Source: three-view drawing plus pictorial views. Frame: mm from the lowest corner of the part. A direction names the side the tool comes from. Round coordinates to 2 decimals unless told otherwise and drop trailing zeros. Loops run counter-clockwise (first coordinate to the right, second up) from the corner with the lowest first, then second, coordinate; pieces in that order, holes last. Notation, with made-up numbers: M 39,57 L 71,57 A13 ccw 71,82 Z; hole C 21.5,19.5 d6. An arc over 180 degrees is marked long. Return JSON: item names as keys, results as strings. Group by question number.
1) Material intervals for line 1 (X direction, y = 15.25, z = 11) (1 decimal); line 2 (Y direction, x = 28.5, z = 9.5); line 3 (Z direction, x = 14.5, y = 16.25), sorted ascending. Write a range as from..to.
2) Access query for the marked faces 4, 5, 6, 7 and 8. Directions: +Z, -Z, +X, -X, +Y, -Y. A direction counts if a zero-diameter tool reaches every point of the face in a straight line with its end or side. Return the directions, or none.
3) Section C-C (x = 7.5). Output: boundary loops of the cut face in (y, z).
4) Section A-A (z = 11). Output: boundary loops of the cut face in (x, y) (1 decimal), plus the area to 3 significant figures.
5) Section D-D (y = 8.75). Output: boundary loops of the cut face in (x, z) (1 decimal), plus the area to 3 significant figures.
6) Section B-B (z = 2.5). Output: boundary loops of the cut face in (x, y) (1 decimal), plus the area to 3 significant figures.
7) Contact query for flat-ended pins moving along their axis: P1, Ø9, axis at x = 24.74, z = 11, coming from the -Y side; P2, Ø5.5, axis at y = 17, z = 20, coming from the +X side; P3, Ø2, axis at y = 11.5, z = 20, coming from the -X side; P4, Ø1.5, axis at x = 43.5, z = 9, coming from the -Y side. Output: stop coordinate, or through.
8) Mould query, pull axis X, two halves, no side actions, for the marked faces 1, 2 and 3. Classes: +X half, -X half, draft (parallel to the pull), parting line (faces both ways), or undercut.
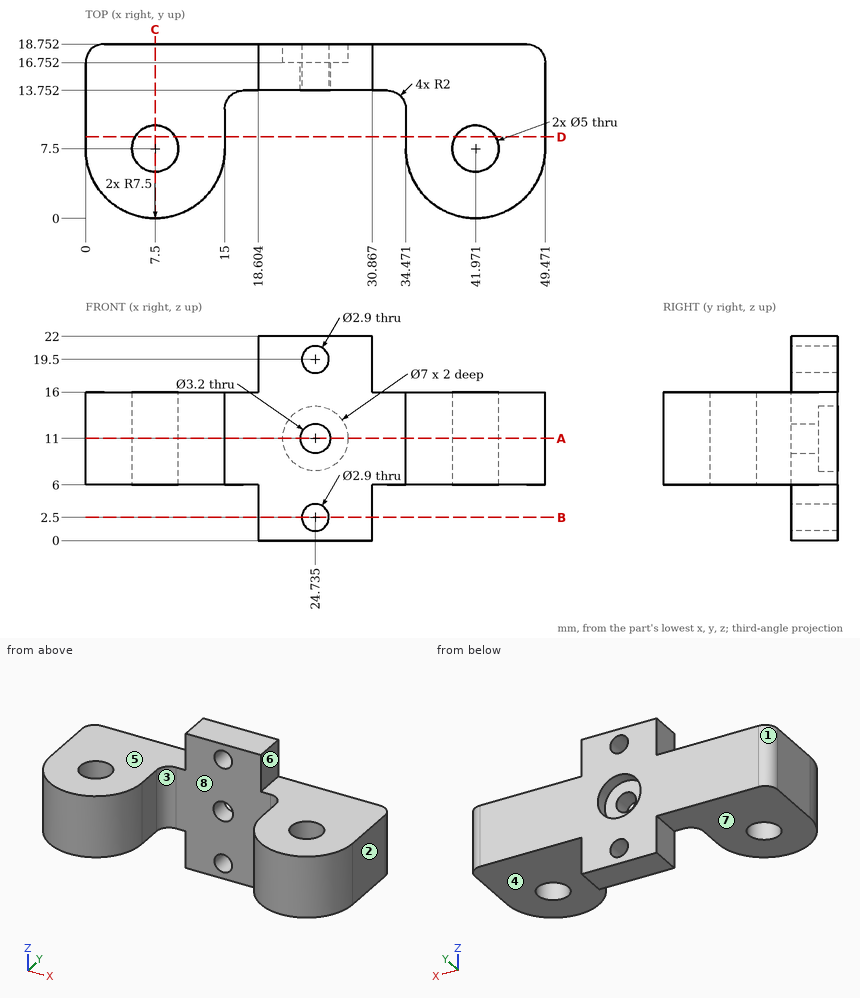
Returned:
{
 "1": {"line 1": "x = 0..23.1, 26.3..49.5", "line 2": "y = 13.75..18.75", "line 3": "z = 6..16"},
 "2": {"face 4": "-Z, +X, +Y, -Y", "face 5": "+Z, -X, +Y, -Y", "face 6": "+Z, +X, +Y, -Y", "face 7": "-Z, -X, +Y, -Y", "face 8": "+Z, -Z, -Y"},
 "3": {"outline": "M 0,6 L 5,6 L 5,16 L 0,16 Z; M 10,6 L 18.75,6 L 18.75,16 L 10,16 Z"},
 "4": {"outline": "M 0,7.5 A7.5 ccw 15,7.5 L 15,11.8 A2 cw 17,13.8 L 23.1,13.8 L 23.1,16.8 L 21.2,16.8 L 21.2,18.8 L 2,18.8 A2 ccw 0,16.8 Z; M 26.3,13.8 L 32.5,13.8 A2 cw 34.5,11.8 L 34.5,7.5 A7.5 ccw 49.5,7.5 L 49.5,16.8 A2 ccw 47.5,18.8 L 28.2,18.8 L 28.2,16.8 L 26.3,16.8 Z; hole C 7.5,7.5 d5; hole C 42,7.5 d5", "area": "549 mm^2"},
 "5": {"outline": "M 0,6 L 5.3,6 L 5.3,16 L 0,16 Z; M 9.7,6 L 15,6 L 15,16 L 9.7,16 Z; M 34.5,6 L 39.8,6 L 39.8,16 L 34.5,16 Z; M 44.1,6 L 49.5,6 L 49.5,16 L 44.1,16 Z", "area": "213 mm^2"},
 "6": {"outline": "M 18.6,13.8 L 23.3,13.8 L 23.3,18.8 L 18.6,18.8 Z; M 26.2,13.8 L 30.9,13.8 L 30.9,18.8 L 26.2,18.8 Z", "area": "46.8 mm^2"},
 "7": {"P1": "stops at y = 13.75", "P2": "stops at x = 30.87", "P3": "passes through", "P4": "stops at y = 0.04"},
 "8": {"face 1": "-X half", "face 2": "+X half", "face 3": "undercut"}
}
